Verification items for the finished model (mm, model axes). Round coordinates to 2 decimals unless told otherwise and drop trailing zeros. Order: outer loops, then holes, each group sorted by start corner. A loop starts at its lowest first (then second) coordinate and runs counter-clockwise, first axis right, second up. Notation, with made-up numbers: M 50.25,18 L 65.25,18 A30 ccw 65.25,42 Z; hole C 63,-16 d6. An arc over 180 degrees is marked long. Use CSV: the item, a comma, the result in double quotes. Start each with the question number.
Q1. Sectioned sample at A-A (x = 0). Enter the section's corners in (y, z), and give its area (3 significant figures).
Q2. Sectioned sample at C-C (z = 13). Enter the section's corners in (x, y).
Q3. Mould release check, pull along Y, two halves, no side actions. Record for faces 1 (the face through (-1, -40, -2)), 2 (the face through (-4.34, -18.71, 0.56)), 3 (the face through (1, 39, 38)), 4 (the face through (-9, -18, -40)): +Y half, -Y half, draft (parallel to the pull), parting line (faces both ways), or undercut.
Q4. Scan lines: line 1 (Y direction, x = 0, z = 3); line 2 (X direction, y = -10, z = 7); line 3 (X direction, y = 0, z = 35). Record each from-to range of solid material in increasing order.
Q5. Sectioned sample at B-B (y = 8.5). Enter the section's corners in (x, z), and give its area (3 significant figures).
```python
from build123d import *

# Parameters (mm, degrees)
F0_W     = 80
F0_H     = 80
F1_DEPTH = 40
F2_R     = 20
F3_DEPTH = 80.001
F4_R     = 5


with BuildPart() as f1:
    # F0 (on Front) → F1 (new body, symmetric)
    with BuildSketch(Plane.XZ):
        Rectangle(F0_W, F0_H)
    extrude(amount=F1_DEPTH, both=True)

    # F2 (on face) → F3 (cut, through all)
    with BuildSketch(Plane.XY.offset(40)):
        with Locations((0, 0.813212)):
            Circle(F2_R)
    extrude(amount=-F3_DEPTH, mode=Mode.SUBTRACT)

    # F4
    f4_edges = [f1.edges().sort_by_distance(p)[0] for p in [
        (-40, 0, 40),
        (0, -40, 40),
        (40, 0, 40),
        (0, 40, 40),
    ]]
    fillet(f4_edges, radius=F4_R)


solid = f1.part
```
Verdict:
1,outline,"M -40,-40 L -19.19,-40 L -19.19,40 L -35,40 A5 ccw -40,35 Z; M 20.81,-40 L 40,-40 L 40,35 A5 ccw 35,40 L 20.81,40 Z"
1,area,"3,190 mm²"
2,outline,"M -40,-40 L 40,-40 L 40,40 L -40,40 Z; hole C 0,0.81 d40"
3,face 1,"-Y half"
3,face 2,"undercut"
3,face 3,"+Y half"
3,face 4,"draft"
4,line 1,"y = -40 to -19.19, 20.81 to 40"
4,line 2,"x = -40 to -16.82, 16.82 to 40"
4,line 3,"x = -40 to -19.98, 19.98 to 40"
5,outline,"M -40,-40 L -18.46,-40 L -18.46,40 L -35,40 A5 ccw -40,35 Z; M 18.46,-40 L 40,-40 L 40,35 A5 ccw 35,40 L 18.46,40 Z"
5,area,"3,440 mm²"
